Input: part model. Units: mm. Frame: model coordinates. A direction names the side the tool comes from. Round coordinates to 2 decimals unless told otherwise and drop trailing zeros. Loops run counter-clockwise (first coordinate to the right, second up) from the corner with the lowest first, then second, coordinate; pieces in that order, holes last. Notation, with made-up numbers: (35.25, 13.5) -> (93.25, 13.5) arc R29 ccw to (93.25, 33.5) -> close; hole circle Ø1 at (-14, 33.5). An arc over 180 degrees is marked (long way). Answer as a JSON object with one key per item and string values. Group by question number.
Item 1: Section query A-A on x = -11. Return loops of the section in (y, z) (3 decimals), and give its area (3 significant figures).
Item 2: Section query B-B on x = -16.5. Return loops of the section in (y, z), and give its area (3 significant figures).
Item 3: Pin query (flat end, axial travel): pin 1 (1.5 mm diameter, centred on x = -7, y = 10.5, fed in from +Z); pin 2 (2 mm diameter, centred on x = -13.5, y = 14, fed in from +Z); pin 3 (0.5 mm diameter, centred on y = 16.5, z = 1, fed in from +X); pin 4 (1.8 mm diameter, centred on x = -16.15, y = 8.6, fed in from +Z). Return the tip coordinate at first contact, or that it passes through.
Item 4: Material intervals for line 1 (Z direction, x = -12.25, y = 17.25); line 2 (X direction, y = 11, z = 4); line 3 (Y direction, x = -11.25, z = 1.25), sorted ascending. Write a range as [from, to].
Item 5: Section query D-D on z = 7. Return loops of the section in (x, y).
Item 6: Section query C-C on y = 16.75. Return loops of the section in (x, z), and give its area (3 significant figures).
Item 7: Draft query along Y for faces 6 (the flat face through (-8.38, 8.104, 0.813)), 7 (the cylindrical face through (-10.556, 12.304, 8.799)), 8 (the flat face through (-12.69, 16, 1)). Return one class per face: released by +Y, released by -Y, zero draft, split by the parting line, or undercut.
Item 8: Set-up query: faces 1 (the cylindrical face through (-10.02, 13.15, 8.95)), 2 (the cylindrical face through (-13.188, 11.64, 2.564)), 3 (the flat face through (-9.39, 16, 1)), 4 (the cylindrical face through (-11.85, 18.19, 0.81)), 5 (the flat face through (-15, 9.4, 1.65)). Return all of +Z, -Z, +X, -X, +Y, -Y with unobstructed straight access to the full face (end or side cutting, diameter ignored); none if empty.
from build123d import *

# Parameters (mm, degrees)
F0_R     = 1.1
F0_R_2   = 2.15
F1_DEPTH = 1.65
F2_R     = 2.75
F2_R_2   = 2.15
F3_DEPTH = 3.85
F4_R     = 2.15
F4_R_2   = 1.9
F4_R_3   = 0.9
F5_DEPTH = 0.3
F6_DEPTH = 7


with BuildPart() as f1:
    # F0 (on Top) → F1 (new body)
    with BuildSketch(Plane.XY):
        with BuildLine():
            ThreePointArc((-12.690082, 13.745292), (-11.040082, 14.295292), (-9.390082, 13.745292))
            Line((-9.390082, 13.745292), (-9.390082, 17.445292))
            ThreePointArc((-9.390082, 17.445292), (-11.040082, 19.095292), (-12.690082, 17.445292))
            Line((-12.690082, 17.445292), (-12.690082, 13.745292))
        make_face()
        with Locations((-11.040082, 17.445292)):
            Circle(F0_R, mode=Mode.SUBTRACT)
        with BuildLine():
            ThreePointArc((-9.959826, 9.01635), (-8.745174, 10.03007), (-8.290082, 11.545292))
            ThreePointArc((-8.290082, 11.545292), (-8.295022, 11.710059), (-8.309826, 11.874234))
            ThreePointArc((-8.309826, 11.874234), (-8.658512, 12.920292), (-9.390082, 13.745292))
            ThreePointArc((-9.390082, 13.745292), (-11.040082, 14.295292), (-12.690082, 13.745292))
            ThreePointArc((-12.690082, 13.745292), (-13.421652, 12.920292), (-13.770338, 11.874234))
            ThreePointArc((-13.770338, 11.874234), (-13.421652, 10.170292), (-12.120338, 9.01635))
            ThreePointArc((-12.120338, 9.01635), (-11.040082, 8.795292), (-9.959826, 9.01635))
        make_face()
        with Locations((-11.040082, 11.545292)):
            Circle(F0_R_2, mode=Mode.SUBTRACT)
        with BuildLine():
            ThreePointArc((-8.309826, 11.874234), (-8.295022, 11.710059), (-8.290082, 11.545292))
            ThreePointArc((-8.290082, 11.545292), (-8.745174, 10.03007), (-9.959826, 9.01635))
            Line((-9.959826, 9.01635), (-6.755532, 7.16635))
            ThreePointArc((-6.755532, 7.16635), (-4.50159, 7.770292), (-5.105532, 10.024234))
            Line((-5.105532, 10.024234), (-8.309826, 11.874234))
        make_face()
        with Locations((-5.930532, 8.595292)):
            Circle(F0_R, mode=Mode.SUBTRACT)
        with BuildLine():
            Line((-15.324632, 7.16635), (-12.120338, 9.01635))
            ThreePointArc((-12.120338, 9.01635), (-13.421652, 10.170292), (-13.770338, 11.874234))
            Line((-13.770338, 11.874234), (-16.974632, 10.024234))
            ThreePointArc((-16.974632, 10.024234), (-17.578574, 7.770292), (-15.324632, 7.16635))
        make_face()
        with Locations((-16.149632, 8.595292)):
            Circle(F0_R, mode=Mode.SUBTRACT)
    extrude(amount=F1_DEPTH)

    # F2 (on face) → F3 (join)
    with BuildSketch(Plane.XY.offset(1.65)):
        with Locations((-11.040082, 11.545292)):
            Circle(F2_R)
        with Locations((-11.040082, 11.545292)):
            Circle(F2_R_2, mode=Mode.SUBTRACT)
    extrude(amount=F3_DEPTH)

    # F4 (on face) → F5 (join)
    with BuildSketch(Plane.XY.offset(5.5)):
        with Locations((-11.040082, 11.545292)):
            Circle(F4_R)
        with Locations((-11.040082, 11.545292)):
            Circle(F4_R_2, mode=Mode.SUBTRACT)
        with Locations((-11.040082, 11.545292)):
            Circle(F4_R_2)
        with Locations((-11.040082, 11.545292)):
            Circle(F4_R_3, mode=Mode.SUBTRACT)
    extrude(amount=-F5_DEPTH)

    # F4 (on face) → F6 (join)
    with BuildSketch(Plane.XY.offset(5.5)):
        with Locations((-11.040082, 11.545292)):
            Circle(F4_R_2)
        with Locations((-11.040082, 11.545292)):
            Circle(F4_R_3, mode=Mode.SUBTRACT)
    extrude(amount=F6_DEPTH)


solid = f1.part
Solved:
{
 "1": {"outline": "(8.796, 0) -> (9.396, 0) -> (9.396, 5.2) -> (10.646, 5.2) -> (10.646, 12.5) -> (9.646, 12.5) -> (9.646, 5.5) -> (8.796, 5.5) -> close; (12.444, 5.2) -> (13.695, 5.2) -> (13.695, 0) -> (16.346, 0) -> (16.346, 1.65) -> (14.295, 1.65) -> (14.295, 5.5) -> (13.445, 5.5) -> (13.445, 12.5) -> (12.444, 12.5) -> close; (18.545, 0) -> (19.095, 0) -> (19.095, 1.65) -> (18.545, 1.65) -> close", "area": "25.6 mm²"},
 "2": {"outline": "(6.98, 0) -> (7.55, 0) -> (7.55, 1.65) -> (6.98, 1.65) -> close; (9.64, 0) -> (10.3, 0) -> (10.3, 1.65) -> (9.64, 1.65) -> close", "area": "2.03 mm²"},
 "3": {"pin 1": "z = 1.65", "pin 2": "z = 5.5", "pin 3": "x = -9.39", "pin 4": "through"},
 "4": {"line 1": "[0, 1.65]", "line 2": "[-13.74, -13.12], [-8.96, -8.34]", "line 3": "[8.8, 9.41], [13.69, 16.37], [18.53, 19.08]"},
 "5": {"outline": "circle Ø3.8 at (-11.04, 11.55); hole circle Ø1.8 at (-11.04, 11.55)"},
 "6": {"outline": "(-12.69, 0) -> (-11.89, 0) -> (-11.89, 1.65) -> (-12.69, 1.65) -> close; (-10.19, 0) -> (-9.39, 0) -> (-9.39, 1.65) -> (-10.19, 1.65) -> close", "area": "2.63 mm²"},
 "7": {"face 6": "released by -Y", "face 7": "undercut", "face 8": "zero draft"},
 "8": {"face 1": "+Z", "face 2": "-Z", "face 3": "+Z, -Z, +X, +Y", "face 4": "+Z, -Z", "face 5": "+Z, -X, -Y"}
}
